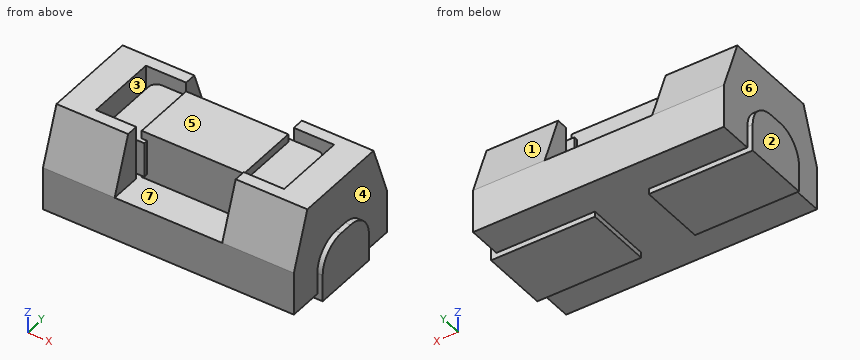
from build123d import *
from OCP.BRepFilletAPI import BRepFilletAPI_MakeChamfer

# Parameters (mm, degrees)
BOSS_EXTRUDE1_START  = 0.2
SKETCH1_W            = 9.33
SKETCH1_H            = 5.03
BOSS_EXTRUDE1_DEPTH  = 3.61
CUT_EXTRUDE1_DEPTH   = 2
CHAMFER1_SIZE        = 2
CHAMFER1_SIZE2       = 0.727940469
BOSS_EXTRUDE3_DEPTH  = 1.25
FILLET2_R            = 1
FILLET2_OF_MIRROR1_R = 1
BOSS_EXTRUDE4_START  = 0.2
SKETCH7_W            = 1.5
SKETCH7_H            = 2.7
BOSS_EXTRUDE4_DEPTH  = 1.3
FILLET3_R            = 0.3
BOSS_EXTRUDE5_START  = -1.49
SKETCH8_W            = 3.8
SKETCH8_H            = 2.4
BOSS_EXTRUDE5_DEPTH  = 1.79


with BuildPart() as part:
    # Sketch1 → Boss-Extrude1 (new body)
    with BuildSketch(Plane.XY.offset(BOSS_EXTRUDE1_START)):
        Rectangle(SKETCH1_W, SKETCH1_H)
    extrude(amount=BOSS_EXTRUDE1_DEPTH)

    # Sketch2 → Cut-Extrude1 (cut)
    with BuildSketch(Plane.XY.offset(3.81)):
        Polygon((-3.5, 1.35), (-2, 1.35), (-2, 2.515), (2, 2.515), (2, 1.35), (3.5, 1.35), (3.5, -1.35), (2, -1.35), (2, -2.515), (-2, -2.515), (-2, -1.35), (-3.5, -1.35), align=None)
    extrude(amount=-CUT_EXTRUDE1_DEPTH, mode=Mode.SUBTRACT)

    # Chamfer1: one chamfer whose edges measure the first distance from different faces: ONE call of the kernel's chamfer builder (chamfer() names one face for all edges)
    chamfer1_edges_1 = [part.edges().sort_by_distance(p)[0] for p in [
        (-3.3325, 2.515, 3.81),
        (3.3325, 2.515, 3.81),
    ]]
    chamfer1_side_1 = [part.faces().sort_by_distance(p)[0] for p in [
        (0, 2.515, 1.754233878),
    ]]
    chamfer1_edges_2 = [part.edges().sort_by_distance(p)[0] for p in [
        (3.3325, -2.515, 3.81),
        (-3.3325, -2.515, 3.81),
    ]]
    chamfer1_side_2 = [part.faces().sort_by_distance(p)[0] for p in [
        (0, -2.515, 1.754233878),
    ]]
    chamfer1 = BRepFilletAPI_MakeChamfer(part.part.solid().wrapped)
    for e in chamfer1_edges_1:
        chamfer1.Add(CHAMFER1_SIZE, CHAMFER1_SIZE2, e.wrapped, chamfer1_side_1[0].wrapped)  # the first distance lies on this face
    for e in chamfer1_edges_2:
        chamfer1.Add(CHAMFER1_SIZE, CHAMFER1_SIZE2, e.wrapped, chamfer1_side_2[0].wrapped)  # the first distance lies on this face
    add(Compound.cast(chamfer1.Shape()), mode=Mode.REPLACE)

    # Sketch6 → Boss-Extrude3 (add, symmetric)
    with BuildSketch(Plane(origin=(0, 0, 0), x_dir=(1, 0, 0), z_dir=(0, 1, 0))):
        Polygon((4.665, -2), (4.865, -2), (4.865, 0), (1, 0), (1, -0.2), (4.665, -0.2), align=None)
    boss_extrude3 = extrude(amount=BOSS_EXTRUDE3_DEPTH, both=True)

    # Fillet2
    fillet2_edges = [part.edges().sort_by_distance(p)[0] for p in [
        (4.765, -1.25, 2),
        (4.765, 1.25, 2),
    ]]
    fillet(fillet2_edges, radius=FILLET2_R)

    # Mirror1: Boss-Extrude3 across plane
    add(boss_extrude3.mirror(Plane(origin=(0, 0, 0), x_dir=(0, 0, 1), z_dir=(1, 0, 0))))

    # Fillet2 of Mirror1
    fillet2_of_mirror1_edges = [part.edges().sort_by_distance(p)[0] for p in [
        (-4.765, -1.25, 2),
        (-4.765, 1.25, 2),
    ]]
    fillet(fillet2_of_mirror1_edges, radius=FILLET2_OF_MIRROR1_R)



with BuildPart() as body_2:
    # Sketch7 → Boss-Extrude4 (new body)
    with BuildSketch(Plane.XY.offset(1.81).offset(BOSS_EXTRUDE4_START)):
        with Locations((-2.45, 0)):
            Rectangle(SKETCH7_W, SKETCH7_H)
    extrude(amount=BOSS_EXTRUDE4_DEPTH)

    # Fillet3
    fillet3_edges = [body_2.edges().sort_by_distance(p)[0] for p in [
        (-3.2, 1.35, 2.66),
        (-3.2, -1.35, 2.66),
    ]]
    fillet(fillet3_edges, radius=FILLET3_R)


with BuildPart() as body_3:
    # Mirror2: mirrored copy
    add(body_2.part.mirror(Plane(origin=(0, 0, 0), x_dir=(0, 0, 1), z_dir=(1, 0, 0))))


with BuildPart() as part_1:
    add(part.part)

    add(body_2.part)  # Boss-Extrude5 merges body 2

    add(body_3.part)  # Boss-Extrude5 merges body 3
    # Sketch8 → Boss-Extrude5 (add)
    with BuildSketch(Plane.XY.offset(3.31).offset(BOSS_EXTRUDE5_START)):
        Rectangle(SKETCH8_W, SKETCH8_H)
    extrude(amount=BOSS_EXTRUDE5_DEPTH)


solid = part_1.part
Model file for the job. Use its own axes, mm. Face numbers are marked on the shaded views. A direction names the side the tool comes from. Coordinates: 2 decimals unless noted, no trailing zeros. Write each loop counter-clockwise with the first axis right and the second up, starting at its lowest first coordinate (ties: lowest second). Pieces come first, ordered by that corner, then holes. Notation, with made-up numbers: (75, 55.25) - (119, 55.25) arc R29 cw to (119, 91.25) - close; hole circle Ø11 at (16, 58). An arc over 180 degrees is marked (long way). Write each question's results on one line, items separated by ' | '. Start each with the question number.
1) Flat gauge pins, fed straight in: P1, Ø1.6, axis at y = 0.5, z = 3, coming from the +X side (3 decimals); P2, Ø1.3, axis at y = -2, z = 3, coming from the -X side (3 decimals); P3, Ø0.8, axis at x = 2.5, y = 0, coming from the +Z side. Where does each tip first touch, or does it go through?
2) Cut at B-B (x = 0.5). Write the cut outline in (y, z) (3 decimals).
3) 3-axis set-ups, long thin cutter, end or side, ignore diameter. For the marked faces 4, 5, 6 and 7: which of +Z, -Z, +X, -X, +Y, -Y reach the whole face in a straight line?
4) Probe line 1 along X through (y, z) = (-0.9, 3) (3 decimals); line 2 along X through (y, z) = (-0.2, 3.35) (3 decimals); line 3 along X through (y, z) = (-2.05, 2.7) (3 decimals). List the from-to ranges inside material, lowest first. Write a range as from..to.
5) Mould opens along X. For the marked faces 1, 2 and 3 say: pulls with the +X half, pulls with the -X half, needs draft (parallel to the pull), parting line crosses it, or undercut.
6) Cut at A-A (y = 0). Write the cut outline in (x, z) (3 decimals), then the cut area to 3 significant figures.
7) Cut at C-C (z = 0.85). Write the cut outline in (x, y) (3 decimals).
8) Cut at D-D (x = 2.5). Write the cut outline in (y, z) (3 decimals), then the cut area to 3 significant figures.
Returned:
1) P1: x = 4.665 | P2: x = -4.665 | P3: z = 3.31
2) outline: (-2.515, 0.2) - (2.515, 0.2) - (2.515, 1.81) - (-2.515, 1.81) - close; (-1.2, 1.82) - (1.2, 1.82) - (1.2, 3.61) - (-1.2, 3.61) - close
3) face 4: +Z, +X | face 5: +Z, +Y, -Y | face 6: +Z, -X | face 7: none
4) line 1: -4.665..-3.5, -3.2..3.2, 3.5..4.665 | line 2: -4.665..-3.5, -1.9..1.9, 3.5..4.665 | line 3: -4.665..-2, 2..4.665
5) face 1: needs draft | face 2: pulls with the -X half | face 3: undercut
6) outline: (-4.865, 0) - (-1, 0) - (-1, 0.2) - (1, 0.2) - (1, 0) - (4.865, 0) - (4.865, 2) - (4.665, 2) - (4.665, 3.81) - (3.5, 3.81) - (3.5, 1.81) - (-3.5, 1.81) - (-3.5, 3.81) - (-4.665, 3.81) - (-4.665, 2) - (-4.865, 2) - close; (-3.2, 2.01) - (-1.9, 2.01) - (-1.9, 1.82) - (1.9, 1.82) - (1.9, 2.01) - (3.2, 2.01) - (3.2, 3.31) - (1.9, 3.31) - (1.9, 3.61) - (-1.9, 3.61) - (-1.9, 3.31) - (-3.2, 3.31) - close | area: 32.1 mm^2
7) outline: (-4.865, -1.25) - (-4.665, -1.25) - (-4.665, -2.515) - (4.665, -2.515) - (4.665, -1.25) - (4.865, -1.25) - (4.865, 1.25) - (4.665, 1.25) - (4.665, 2.515) - (-4.665, 2.515) - (-4.665, 1.25) - (-4.865, 1.25) - close
8) outline: (-2.515, 0.2) - (-1.25, 0.2) - (-1.25, 0) - (1.25, 0) - (1.25, 0.2) - (2.515, 0.2) - (2.515, 1.81) - (1.787, 3.81) - (1.35, 3.81) - (1.35, 3.31) - (-1.35, 3.31) - (-1.35, 3.81) - (-1.787, 3.81) - (-2.515, 1.81) - close; hole (-1.35, 1.81) - (1.35, 1.81) - (1.35, 2.01) - (-1.35, 2.01) - close | area: 15.3 mm^2
